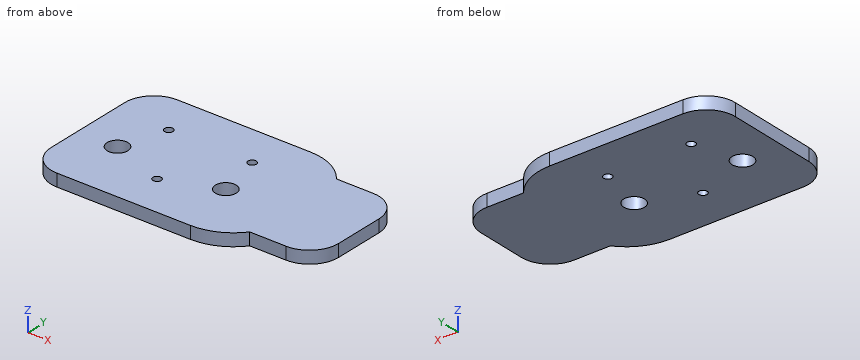
from build123d import *

# Parameters (mm, degrees)
INSERT_IN_SHEET_METAL_HOLE_DEPTH = 1
BACKING_DEPTH                    = 3
SCREWHOLES_DEPTH                 = 46.793012567
SCREWHOLES_DEPTH_BACK            = 46.793012567
SKETCH3_R                        = 1
WIRE_HOLES_DEPTH                 = 46.793012567
WIRE_HOLES_DEPTH_BACK            = 46.793012567
SKETCH4_R                        = 2.5


with BuildPart() as part:
    # Sketch1 → Insert in sheet metal hole (new body)
    with BuildSketch(Plane.XY):
        with BuildLine():
            Line((-18, 11), (-18, -11))
            ThreePointArc((-18, -11), (-17.414213562, -12.414213562), (-16, -13))
            Line((-16, -13), (16, -13))
            ThreePointArc((16, -13), (20, -11.92820323), (22.92820323, -9))
            ThreePointArc((22.92820323, -9), (23.660254038, -8.267949192), (24.660254038, -8))
            Line((24.660254038, -8), (35, -8))
            ThreePointArc((35, -8), (36.414213562, -7.414213562), (37, -6))
            Line((37, -6), (37, 6))
            ThreePointArc((37, 6), (36.414213562, 7.414213562), (35, 8))
            Line((35, 8), (24.660254038, 8))
            ThreePointArc((24.660254038, 8), (23.660254038, 8.267949192), (22.92820323, 9))
            ThreePointArc((22.92820323, 9), (20, 11.92820323), (16, 13))
            Line((16, 13), (-16, 13))
            ThreePointArc((-16, 13), (-17.414213562, 12.414213562), (-18, 11))
        make_face()
    extrude(amount=INSERT_IN_SHEET_METAL_HOLE_DEPTH)

    # Sketch2 → Backing (add)
    with BuildSketch(Plane.XY.offset(1)):
        with BuildLine():
            Line((26.246950766, -13), (35, -13))
            ThreePointArc((35, -13), (39.949747468, -10.949747468), (42, -6))
            Line((42, -6), (42, 6))
            ThreePointArc((42, 6), (39.949747468, 10.949747468), (35, 13))
            Line((35, 13), (26.246950766, 13))
            ThreePointArc((26.246950766, 13), (21.700877125, 16.683321446), (16, 18))
            Line((16, 18), (-16, 18))
            ThreePointArc((-16, 18), (-20.949747468, 15.949747468), (-23, 11))
            Line((-23, 11), (-23, -11))
            ThreePointArc((-23, -11), (-20.949747468, -15.949747468), (-16, -18))
            Line((-16, -18), (16, -18))
            ThreePointArc((16, -18), (21.700877125, -16.683321446), (26.246950766, -13))
        make_face()
    extrude(amount=-BACKING_DEPTH)

    # Sketch3 → Screwholes (cut, two sides: drawn at the far end of the back side and taken through both)
    with BuildSketch(Plane.XY.offset(1).offset(-SCREWHOLES_DEPTH_BACK)):
        with Locations((-10, 8)):
            Circle(SKETCH3_R)
        with Locations((10, 8)):
            Circle(SKETCH3_R)
        with Locations((0, -8)):
            Circle(SKETCH3_R)
    extrude(amount=SCREWHOLES_DEPTH + SCREWHOLES_DEPTH_BACK, mode=Mode.SUBTRACT)

    # Sketch4 → Wire holes (cut, two sides: drawn at the far end of the back side and taken through both)
    with BuildSketch(Plane.XY.offset(1).offset(-WIRE_HOLES_DEPTH_BACK)):
        with Locations((-13.5, -3)):
            Circle(SKETCH4_R)
        with Locations((12.5, -3)):
            Circle(SKETCH4_R)
    extrude(amount=WIRE_HOLES_DEPTH + WIRE_HOLES_DEPTH_BACK, mode=Mode.SUBTRACT)


solid = part.part
Could you check a few things on this model? Use its own coordinates, in mm. Give positions to 0.01 mm unless a question says otherwise; leave off trailing zeros. Order: outer loops, then holes, each group sorted by start corner. A loop starts at its lowest first (then second) coordinate and runs counter-clockwise, first axis right, second up. Notation, with made-up numbers: (-32.75, -2) -> (-15.75, -2) arc R31 ccw to (-15.75, 23) -> close; hole circle Ø9 at (12, 73). An arc over 180 degrees is marked (long way). Answer in a Markdown table with one row per item. Add a question column.
Item 1: Please list where these lines run through material, in increasing order: probe 1 along X at (y, z) = (-3, 0); probe 2 along Y at (x, z) = (12.5, 0.8); probe 3 along X at (y, z) = (-1, -0.6).
Item 2: I'm going to push flat-ended pins straight in: P1, Ø4, axis at x = -13.5, y = -3, coming from the +Z side; P2, Ø6.5, axis at x = 12.5, y = -3, coming from the -Z side; P3, Ø1.5, axis at x = 28.5, z = -0.5, coming from the -Y side; P4, Ø1, axis at y = 14, z = -0.5, coming from the -X side. Where does each tip first touch, or does it pass through?
Item 3: Imagine slicing it at B-B (y = -8). List the corners of the cut face in (x, z) for me.
Item 4: Imagine slicing it at C-C (z = -1.4). List the corners of the cut face in (x, y) for me, and give its area (3 significant figures).
Item 5: Imagine slicing it at A-A (x = -13.5). List the corners of the cut face in (y, z) for me.
Item 6: Imagine slicing it at D-D (x = 30). List the corners of the cut face in (y, z) for me.
Result:
| question | item | result |
|---|---|---|
| 1 | probe 1 | -23 to -16, -11 to 10, 15 to 42 |
| 1 | probe 2 | -18 to -5.5, -0.5 to 18 |
| 1 | probe 3 | -23 to -15, -12 to 11, 14 to 42 |
| 2 | P1 | through |
| 2 | P2 | z = -2 |
| 2 | P3 | y = -13 |
| 2 | P4 | x = -22.54 |
| 3 | outline | (-23, -2) -> (-1, -2) -> (-1, 1) -> (-23, 1) -> close; (1, -2) -> (41.71, -2) -> (41.71, 1) -> (1, 1) -> close |
| 4 | outline | (-23, -11) arc R7 ccw to (-16, -18) -> (16, -18) arc R13 ccw to (26.25, -13) -> (35, -13) arc R7 ccw to (42, -6) -> (42, 6) arc R7 ccw to (35, 13) -> (26.25, 13) arc R13 ccw to (16, 18) -> (-16, 18) arc R7 ccw to (-23, 11) -> close; hole circle Ø5 at (-13.5, -3); hole circle Ø2 at (-10, 8); hole circle Ø2 at (0, -8); hole circle Ø2 at (10, 8); hole circle Ø5 at (12.5, -3) |
| 4 | area | 2,060 mm2 |
| 5 | outline | (-18, -2) -> (-5.5, -2) -> (-5.5, 1) -> (-18, 1) -> close; (-0.5, -2) -> (18, -2) -> (18, 1) -> (-0.5, 1) -> close |
| 6 | outline | (-13, -2) -> (13, -2) -> (13, 1) -> (-13, 1) -> close |
